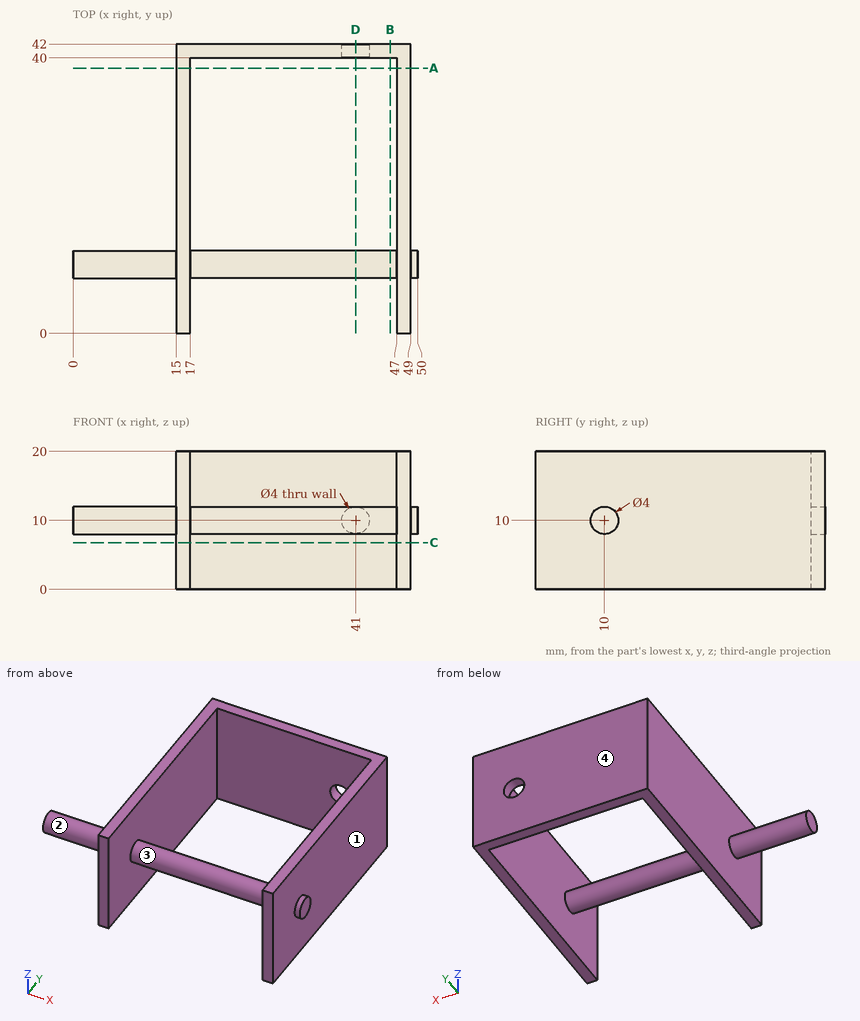
Could you check a few things on this drawing? It's one solid part, dimensions in mm from its lowest x, y, z. Round coordinates to 2 decimals unless told otherwise and drop trailing zeros. Order: outer loops, then holes, each group sorted by start corner. A loop starts at its lowest first (then second) coordinate and runs counter-clockwise, first axis right, second up.
Q1. Thinking about a two-plate mould opening in Y: for the marked faces 1, 2, 3 and 4, which applies, released by +Y, released by -Y, zero draft, split by the parting line, or undercut?
Geometry says:
face 1: zero draft
face 2: split by the parting line
face 3: undercut
face 4: released by +Y
Q2. I'm going to push flat-ended pins straight in: P1, Ø4, axis at y = 28.5, z = 7, coming from the -X side; P2, Ø10, axis at y = 16, z = 10, coming from the +X side; P3, Ø10, axis at x = 30, z = 5, coming from the -Y side; P4, Ø8, axis at y = 20, z = 8.5, coming from the +X side. Where does each tip first touch, or does it pass through?
Geometry says:
P1: stops at x = 15
P2: stops at x = 50
P3: stops at y = 8
P4: stops at x = 49
Q3. Imagine slicing it at D-D, the plane x = 41. List the corners of the cut face in (y, z) for me, then the cut area to 3 significant figures.
Geometry says:
outline: circle Ø4 at (10, 10); (40, 0) - (42, 0) - (42, 8) - (40, 8) - close; (40, 12) - (42, 12) - (42, 20) - (40, 20) - close
area: 44.6 mm2
Q4. Imagine slicing it at A-A, the plane y = 38.5. List the corners of the cut face in (x, z) for me, then the cut area to 3 significant figures.
Geometry says:
outline: (15, 0) - (17, 0) - (17, 20) - (15, 20) - close; (47, 0) - (49, 0) - (49, 20) - (47, 20) - close
area: 80.0 mm2
Q5. Imagine slicing it at C-C, the plane z = 6.75. List the corners of the cut face in (x, y) for me.
Geometry says:
outline: (15, 0) - (17, 0) - (17, 40) - (47, 40) - (47, 0) - (49, 0) - (49, 42) - (15, 42) - close
Q6. Please list where these lines run through material, in increasing order: probe 1 along X at (y, z) = (31, 1.5); probe 2 along X at (y, z) = (41.1, 10); probe 3 along Z at (x, y) = (41, 40.7).
Geometry says:
probe 1: x = 15 to 17, 47 to 49
probe 2: x = 15 to 39, 43 to 49
probe 3: z = 0 to 8, 12 to 20
Q7. Imagine slicing it at B-B, the plane x = 46. List the corners of the cut face in (y, z) for me.
Geometry says:
outline: circle Ø4 at (10, 10); (40, 0) - (42, 0) - (42, 20) - (40, 20) - close
